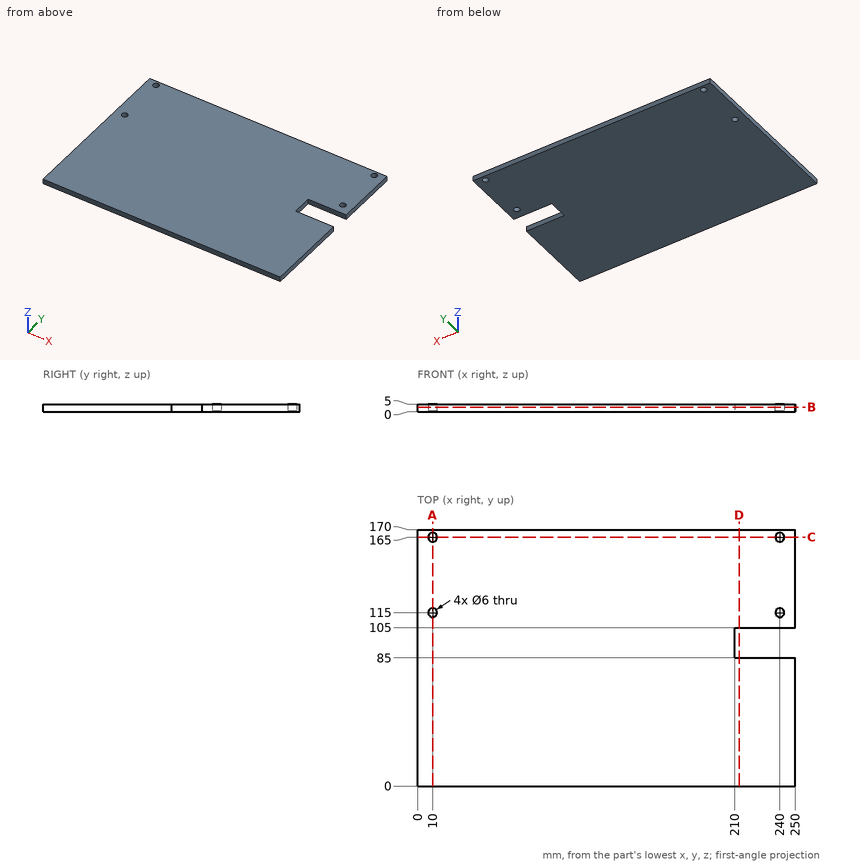
Could you check a few things on this drawing? It's one solid part, dimensions in mm from its lowest x, y, z. Coordinates: 2 decimals unless noted, no trailing zeros. Loops run counter-clockwise (first coordinate to the right, second up) from the corner with the lowest first, then second, coordinate; pieces in that order, holes last.
1. Imagine slicing it at B-B (z = 2.9). Please give me the cut outline in (x, y), and give its area (3 significant figures).
2. For P1, Ø3.5, axis at x = 10, y = 115, coming from the +Z side, with a flat end and sliding along its axis, tell me the tip position at first contact or that it passes through.
3. Imagine slicing it at C-C (y = 165). Please give me the cut outline in (x, z), and give its area (3 significant figures).
4. Imagine slicing it at A-A (x = 10). Please give me the cut outline in (y, z), and give its area (3 significant figures).
5. I need wall thicknesses on L1, parallel to X at y = 115, z = 3.1; L2, parallel to Y at x = 240, z = 1.85; L3, parallel to Y at x = 10, z = 3.95. Which ranges of each line are inside material? Lowest first, please.
6. Imagine slicing it at D-D (x = 213). Please give me the cut outline in (y, z).
Computed values:
1. outline: (0, 0) - (250, 0) - (250, 85) - (210, 85) - (210, 105) - (250, 105) - (250, 170) - (0, 170) - close; hole circle Ø6 at (10, 115); hole circle Ø6 at (10, 165); hole circle Ø6 at (240, 115); hole circle Ø6 at (240, 165)
1. area: 41,600 mm2
2. P1: passes through
3. outline: (0, 0) - (7, 0) - (7, 5) - (0, 5) - close; (13, 0) - (237, 0) - (237, 5) - (13, 5) - close; (243, 0) - (250, 0) - (250, 5) - (243, 5) - close
3. area: 1,190 mm2
4. outline: (0, 0) - (112, 0) - (112, 5) - (0, 5) - close; (118, 0) - (162, 0) - (162, 5) - (118, 5) - close; (168, 0) - (170, 0) - (170, 5) - (168, 5) - close
4. area: 790 mm2
5. L1: x = 0 to 7, 13 to 237, 243 to 250
5. L2: y = 0 to 85, 105 to 112, 118 to 162, 168 to 170
5. L3: y = 0 to 112, 118 to 162, 168 to 170
6. outline: (0, 0) - (85, 0) - (85, 5) - (0, 5) - close; (105, 0) - (170, 0) - (170, 5) - (105, 5) - close
